Could you check a few things on this drawing? It's one solid part, dimensions in mm from its lowest x, y, z. Coordinates: 2 decimals unless noted, no trailing zeros. Order: outer loops, then holes, each group sorted by start corner. A loop starts at its lowest first (then second) coordinate and runs counter-clockwise, first axis right, second up. Notation, with made-up numbers: (-3, 50.5) - (47, 50.5) arc R25 cw to (47, 87.5) - close; hole circle Ø7 at (59, -22.5). An arc over 180 degrees is marked (long way). Answer in a Markdown table with one row per item. Add a question column.
Item 1: Thinking about a two-plate mould opening in X: for the marked faces 1, 2 and 3, which applies, +X half, -X half, draft (parallel to the pull), parting line (faces both ways), or undercut?
Item 2: I want a section at B-B (x = 14). Please give me the cut outline in (y, z) (3 decimals), plus the area to 3 significant figures.
Item 3: I want a section at C-C (z = 7). Please give me the cut outline in (x, y) (1 decimal).
Item 4: I want a section at A-A (z = 18). Please give me the cut outline in (x, y) (3 decimals).
Item 5: If I drill on line 1 along Y through (x, z) = (24, 5.5) (3 decimals); line 2 along X through (y, z) = (10, 19); line 3 along Z through (x, y) = (11, 7.5), over which ranges is the centre line in solid material (lowest first)? Write a range as from..to.
Item 6: I want a section at D-D (x = 9). Please give me the cut outline in (y, z) (3 decimals), plus the area to 3 significant figures.
Item 7: Will these pins go through, and if not, where does the flat tip stop? pin 1 Ø8 at (x, z) = (15.5, 14) entering from +Y; pin 2 Ø12 at (x, y) = (24, 10) entering from +Z; pin 3 Ø4 at (x, y) = (4, 6) entering from +Z; pin 4 Ø2 at (x, y) = (15, 31) entering from +Z.
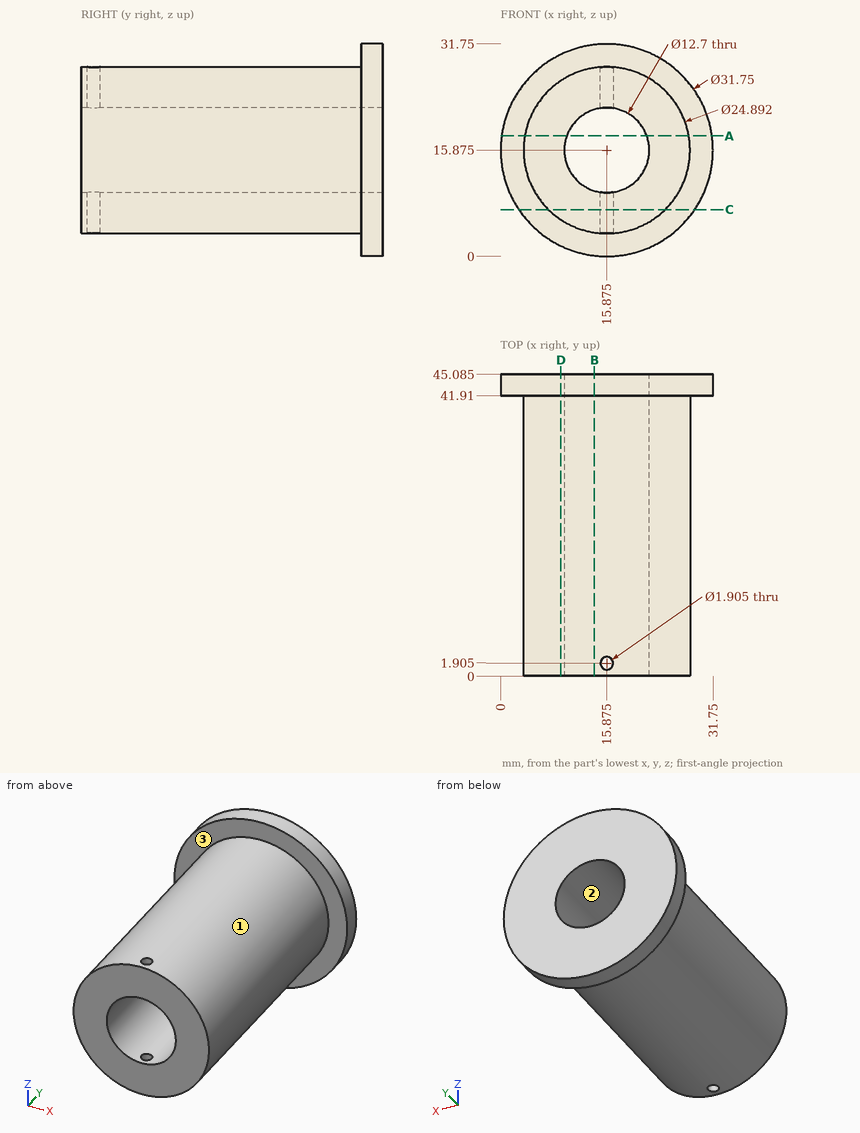
Values follow:
| question | item | result |
|---|---|---|
| 1 | face 1 | parting line |
| 1 | face 2 | undercut |
| 1 | face 3 | draft |
| 2 | outline | (0, 3.571) - (41.91, 3.571) - (41.91, 0.111) - (45.085, 0.111) - (45.085, 9.808) - (0, 9.808) - close; (0, 21.942) - (45.085, 21.942) - (45.085, 31.639) - (41.91, 31.639) - (41.91, 28.179) - (0, 28.179) - close |
| 2 | area | 584 mm^2 |
| 3 | outline | (2.7, 41.9) - (7.1, 41.9) - (7.1, 0) - (24.6, 0) - (24.6, 41.9) - (29, 41.9) - (29, 45.1) - (2.7, 45.1) - close; hole circle Ø1.9 at (15.9, 1.9) |
| 4 | outline | (0.143, 41.91) - (3.612, 41.91) - (3.612, 0) - (9.891, 0) - (9.891, 45.085) - (0.143, 45.085) - close; (21.859, 0) - (28.138, 0) - (28.138, 41.91) - (31.607, 41.91) - (31.607, 45.085) - (21.859, 45.085) - close |
| 5 | line 1 | y = 41.91..45.085 |
| 5 | line 2 | x = 3.83..10.35, 21.4..27.92 |
| 5 | line 3 | z = 4.42..11.81, 19.94..27.33 |
| 6 | outline | (0, 5.5) - (41.91, 5.5) - (41.91, 1.566) - (45.085, 1.566) - (45.085, 30.184) - (41.91, 30.184) - (41.91, 26.25) - (0, 26.25) - close |
| 6 | area | 960 mm^2 |
| 7 | pin 1 | passes through |
| 7 | pin 2 | stops at z = 28.14 |
| 7 | pin 3 | stops at z = 23.45 |
| 7 | pin 4 | stops at z = 28.32 |
